Input: part model. Units: mm. Frame: model coordinates. Face numbers are marked on the shaded views. Round coordinates to 2 decimals unless told otherwise and drop trailing zeros. Loops run counter-clockwise (first coordinate to the right, second up) from the corner with the lowest first, then second, coordinate; pieces in that order, holes last. Notation, with made-up numbers: (22.5, -14.75) -> (80.5, -14.75) arc R28 ccw to (80.5, 10.25) -> close; hole circle Ø7 at (-16, 33.25). An arc over 180 degrees is marked (long way). Answer in a Markdown table with one row per item. Add a question column.
Q1. Section A-A, the plane y = 60. Output: boundary loops of the cut face in (x, z) (3 decimals), and give its area (3 significant figures).
Q2. Section D-D, the plane y = 51.5. Output: boundary loops of the cut face in (x, z) (3 decimals), and give its area (3 significant figures).
Q3. Section C-C, the plane z = 2. Output: boundary loops of the cut face in (x, y).
Q4. Section B-B, the plane x = 101. Output: boundary loops of the cut face in (y, z) (3 decimals).
Q5. Pin query (flat end, axial travel): pin 1 (1 mm diameter, centred on x = 92.5, y = 41, fed in from -Z); pin 2 (2 mm diameter, centred on y = 58.5, z = -2, fed in from -X); pin 3 (1.5 mm diameter, centred on x = 111, z = -1, fed in from -Y). Return the tip coordinate at first contact, or that it passes through.
Q6. Ray query, L1, parallel to X at y = 52.5, z = 1.5; L2, parallel to Y at x = 105, z = 0.75; L3, parallel to Y at x = 104, z = 2.5. Return the intervals inside material, ascending. Write a range as from..to.
Q7. Mould query, pull axis Y, two halves, no side actions, for the marked faces 1 and 2. Classes: pulls with the +Y half, pulls with the -Y half, needs draft (parallel to the pull), parting line crosses it, or undercut.
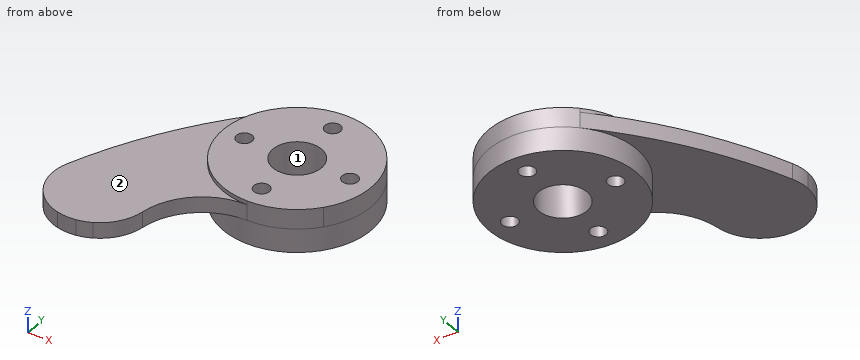
```python
from build123d import *
from build123d.topology import SkipClean

# Parameters (mm, degrees)
SKETCH1_R           = 12
BOSS_EXTRUDE1_DEPTH = 3.175
BOSS_EXTRUDE2_START = 3.81
SKETCH2_R           = 12
BOSS_EXTRUDE2_DEPTH = 3.81
SKETCH3_R           = 3.937
CUT_EXTRUDE1_DEPTH  = 134.099089527
SKETCH4_R           = 1.27
CUT_EXTRUDE2_DEPTH  = 134.099089527
CUT_EXTRUDE3_DEPTH  = 133.970273023
CUT_EXTRUDE4_START  = -0.635
CUT_EXTRUDE4_DEPTH  = 0.635


with BuildPart() as part:
    # Sketch1 → Boss-Extrude1 (new body)
    with BuildSketch(Plane.XY):
        with BuildLine():
            ThreePointArc((79.156979953, 34.616777747), (78.764409425, 33.207913627), (78.648230314, 31.75))
            Line((78.648230314, 31.75), (93.886132052, 31.75))
            ThreePointArc((93.886132052, 31.75), (93.886918896, 31.813218964), (93.887181183, 31.876442281))
            ThreePointArc((93.887181183, 31.876442281), (87.66085737, 39.367908538), (79.156979953, 34.616777747))
        make_face()
        with BuildLine():
            ThreePointArc((87.4395, 24.347161532), (88.598049964, 24.621688616), (89.699693339, 25.073335615))
            ThreePointArc((89.699693339, 25.073335615), (92.723044454, 27.828451492), (93.886132052, 31.75))
            Line((93.886132052, 31.75), (78.648230314, 31.75))
            ThreePointArc((78.648230314, 31.75), (79.141141445, 29.177561465), (80.476005529, 26.924))
            Line((80.476005529, 26.924), (87.4395, 26.924))
            Line((87.4395, 26.924), (87.4395, 24.347161532))
        make_face()
        with BuildLine():
            Line((87.4395, 26.924), (80.476005529, 26.924))
            ThreePointArc((80.476005529, 26.924), (82.246043304, 25.403819152), (84.393093646, 24.490496444))
            ThreePointArc((84.393093646, 24.490496444), (85.909052633, 24.264862685), (87.4395, 24.347161532))
            Line((87.4395, 24.347161532), (87.4395, 26.924))
        make_face()
        with BuildLine():
            ThreePointArc((89.699693339, 25.073335615), (94.483227873, 27.711788353), (99.06, 30.694537484))
            Line((99.06, 30.694537484), (99.06, 31.75))
            Line((99.06, 31.75), (93.886132052, 31.75))
            ThreePointArc((93.886132052, 31.75), (92.723044454, 27.828451492), (89.699693339, 25.073335615))
        make_face()
        with BuildLine():
            ThreePointArc((99.06, 30.694537484), (106.888760949, 37.054762789), (113.784062988, 44.416608597))
            ThreePointArc((113.784062988, 44.416608597), (96.436063978, 43.110085278), (96.014300162, 60.502100346))
            ThreePointArc((96.014300162, 60.502100346), (86.225733854, 48.445051897), (79.156979953, 34.616777747))
            ThreePointArc((79.156979953, 34.616777747), (87.66085737, 39.367908538), (93.887181183, 31.876442281))
            ThreePointArc((93.887181183, 31.876442281), (93.886918896, 31.813218964), (93.886132052, 31.75))
            Line((93.886132052, 31.75), (99.06, 31.75))
            Line((99.06, 31.75), (99.06, 30.694537484))
        make_face()
        with Locations((104.48925, 52.0065)):
            Circle(SKETCH1_R)
    extrude(amount=BOSS_EXTRUDE1_DEPTH)

    # Sketch2 → Boss-Extrude2 (add)
    with SkipClean():  # the faces are left unmerged after this step: merging them gives an invalid solid
        with BuildSketch(Plane(origin=(0, 0, 0), x_dir=(-1, 0, 0), z_dir=(0, 0, -1)).offset(BOSS_EXTRUDE2_START)):
            with Locations((-104.48925, 52.0065)):
                Circle(SKETCH2_R)
        extrude(amount=-BOSS_EXTRUDE2_DEPTH)

    # Sketch3 → Cut-Extrude1 (cut, through all)
    with SkipClean():  # the faces are left unmerged after this step: merging them gives an invalid solid
        with BuildSketch(Plane(origin=(0, 0, -3.81), x_dir=(-1, 0, 0), z_dir=(0, 0, -1))):
            with Locations((-104.48925, 52.0065)):
                Circle(SKETCH3_R)
        extrude(amount=-CUT_EXTRUDE1_DEPTH, mode=Mode.SUBTRACT)

    # Sketch4 → Cut-Extrude2 (cut, through all)
    with SkipClean():  # the faces are left unmerged after this step: merging them gives an invalid solid
        with BuildSketch(Plane(origin=(0, 0, -3.81), x_dir=(-1, 0, 0), z_dir=(0, 0, -1))):
            with Locations((-112.99825, 52.0065)):
                Circle(SKETCH4_R)
            with Locations((-95.98025, 52.0065)):
                Circle(SKETCH4_R)
            with Locations((-104.48925, 60.5155)):
                Circle(SKETCH4_R)
            with Locations((-104.48925, 43.4975)):
                Circle(SKETCH4_R)
        extrude(amount=-CUT_EXTRUDE2_DEPTH, mode=Mode.SUBTRACT)

    # Sketch5 → Cut-Extrude3 (cut, through all)
    with SkipClean():  # the faces are left unmerged after this step: merging them gives an invalid solid
        with BuildSketch(Plane(origin=(0, 0, 0), x_dir=(-1, 0, 0), z_dir=(0, 0, -1))):
            with BuildLine():
                ThreePointArc((-104.430493989, 40.006643845), (-109.606684651, 41.15238269), (-113.7840634, 44.4166091))
                ThreePointArc((-113.7840634, 44.4166091), (-102.758092767, 33.479680706), (-89.699693406, 25.073335649))
                ThreePointArc((-89.699693406, 25.073335649), (-92.462895691, 27.440507008), (-93.81346398, 30.819079549))
                ThreePointArc((-93.81346398, 30.819079549), (-97.397477458, 37.40567327), (-104.430493989, 40.006643845))
            make_face()
        extrude(amount=-CUT_EXTRUDE3_DEPTH, mode=Mode.SUBTRACT)
    add(part.part.scale(1), mode=Mode.REPLACE)  # the faces are merged on a copy

    # Sketch6 → Cut-Extrude4 (cut)
    with BuildSketch(Plane.XY.offset(3.175).offset(CUT_EXTRUDE4_START)):
        with BuildLine():
            ThreePointArc((96.014299675, 60.502099861), (86.225733771, 48.44505177), (79.156980092, 34.616778107))
            ThreePointArc((79.156980092, 34.616778107), (84.355854315, 24.500045491), (93.81346398, 30.819079549))
            ThreePointArc((93.81346398, 30.819079549), (97.397477458, 37.40567327), (104.430493989, 40.006643845))
            ThreePointArc((104.430493989, 40.006643845), (93.388711037, 47.448207038), (96.014299675, 60.502099861))
        make_face()
    extrude(amount=CUT_EXTRUDE4_DEPTH, mode=Mode.SUBTRACT)


solid = part.part
```
Answer block:
| question | item | result |
|---|---|---|
| 1 | outline | (95.516, 0) -> (95.539, 0) -> (95.539, -3.81) -> (103.329, -3.81) -> (103.329, 3.175) -> (95.539, 3.175) -> (95.539, 2.54) -> (95.516, 2.54) -> close; (105.65, -3.81) -> (113.439, -3.81) -> (113.439, 3.175) -> (105.65, 3.175) -> close |
| 1 | area | 109 mm^2 |
| 2 | outline | (88.326, 0) -> (92.5, 0) -> (92.5, -3.81) -> (94.816, -3.81) -> (94.816, 3.175) -> (92.5, 3.175) -> (92.5, 2.54) -> (88.326, 2.54) -> close; (97.145, -3.81) -> (100.585, -3.81) -> (100.585, 3.175) -> (97.145, 3.175) -> close; (108.394, -3.81) -> (111.834, -3.81) -> (111.834, 3.175) -> (108.394, 3.175) -> close; (114.163, -3.81) -> (116.479, -3.81) -> (116.479, 3.175) -> (114.163, 3.175) -> close |
| 2 | area | 91.0 mm^2 |
| 3 | outline | (79.16, 34.62) arc R7.62 ccw (long way) to (93.81, 30.82) arc R10.67 cw to (104.43, 40.01) arc R12 ccw (long way) to (96.01, 60.5) arc R74.31 ccw to start; hole circle Ø2.54 at (95.98, 52.01); hole circle Ø7.87 at (104.49, 52.01); hole circle Ø2.54 at (104.49, 43.5); hole circle Ø2.54 at (104.49, 60.52); hole circle Ø2.54 at (113, 52.01) |
| 4 | outline | (39.458, 0) -> (40.525, 0) -> (40.525, -3.81) -> (50.183, -3.81) -> (50.183, 3.175) -> (40.525, 3.175) -> (40.525, 2.54) -> (39.458, 2.54) -> close; (53.83, -3.81) -> (63.488, -3.81) -> (63.488, 3.175) -> (53.83, 3.175) -> close |
| 5 | pin 1 | z = 0 |
| 5 | pin 2 | x = 93.82 |
| 5 | pin 3 | y = 41.48 |
| 6 | L1 | 89.06..94.81, 97.15..100.58, 108.4..111.83, 114.17..116.48 |
| 6 | L2 | 40.02..42.33, 44.66..48.1, 55.91..59.35, 61.68..64 |
| 6 | L3 | 40..42.33, 44.67..48.1, 55.91..59.34, 61.69..64 |
| 7 | face 1 | undercut |
| 7 | face 2 | needs draft |
